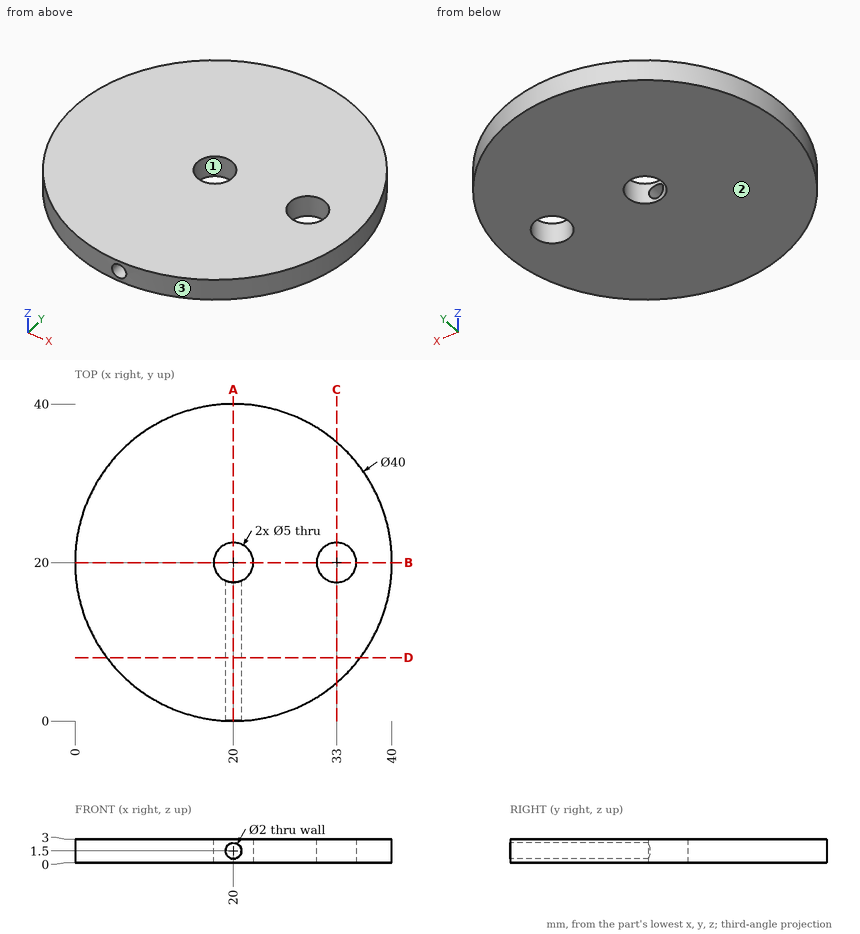
Design review of the part shown in the three views and the two pictorial views. Dimensions are in mm from the part's minimum x, y and z. Coordinates: 2 decimals unless noted, no trailing zeros. Loops run counter-clockwise (first coordinate to the right, second up) from the corner with the lowest first, then second, coordinate; pieces in that order, holes last.
Q1. We need section B-B on y = 20. State the section outline as (x, z) points.
Reported:
outline: (0, 0) - (17.5, 0) - (17.5, 3) - (0, 3) - close; (22.5, 0) - (30.5, 0) - (30.5, 3) - (22.5, 3) - close; (35.5, 0) - (40, 0) - (40, 3) - (35.5, 3) - close
Q2. For pin 1 (1 mm diameter, centred on x = 6.5, z = 2.5, fed in from +Y); pin 2 (1 mm diameter, centred on y = 4.5, z = 2, fed in from -X); pin 3 (1 mm diameter, centred on y = 31.5, z = 2, fed in from -X), all flat-tipped, find the tip position at first contact; note any pin that passes through.
Reported:
pin 1: stops at y = 35.2
pin 2: stops at x = 6.77
pin 3: stops at x = 3.3
Q3. We need section A-A on x = 20. State the section outline as (y, z) points.
Reported:
outline: (0, 0) - (17.5, 0) - (17.5, 0.5) - (0, 0.5) - close; (0, 2.5) - (17.5, 2.5) - (17.5, 3) - (0, 3) - close; (22.5, 0) - (40, 0) - (40, 3) - (22.5, 3) - close
Q4. The part is to be moulded in two halves that separate along Y. For the marked faces 1, 2 and 3, say which applies: +Y half, -Y half, draft (parallel to the pull), parting line (faces both ways), or undercut.
Reported:
face 1: undercut
face 2: draft
face 3: parting line
Q5. To check wall thickness, follow line 1 (X direction, y = 19, z = 0.55); line 2 (Z direction, x = 20, y = 13); line 3 (X direction, y = 22, z = 1.45). State the ranges of each line that lie inside material, in increasing order.
Reported:
line 1: x = 0.03 to 17.71, 22.29 to 30.71, 35.29 to 39.97
line 2: z = 0 to 0.5, 2.5 to 3
line 3: x = 0.1 to 18.5, 21.5 to 31.5, 34.5 to 39.9
Q6. We need section D-D on y = 8. State the section outline as (x, z) points.
Reported:
outline: (4, 0) - (36, 0) - (36, 3) - (4, 3) - close; hole circle Ø2 at (20, 1.5)
Q7. We need section C-C on x = 33. State the section outline as (y, z) points, and give its area (3 significant figures).
Reported:
outline: (4.8, 0) - (17.5, 0) - (17.5, 3) - (4.8, 3) - close; (22.5, 0) - (35.2, 0) - (35.2, 3) - (22.5, 3) - close
area: 76.2 mm2
